from build123d import *

# Parameters (mm, degrees)
BOSS_EXTRUDE2_DEPTH = 100
SKETCH2_W           = 4.5
SKETCH2_H           = 54.5
BOSS_EXTRUDE3_DEPTH = 35
CHAMFER1_SIZE       = 3
DRAFT2_ANGLE        = 4


with BuildPart() as part:
    # Sketch1 → Boss-Extrude2 (new body)
    with BuildSketch(Plane(origin=(0, 0, 0), x_dir=(1, 0, 0), z_dir=(0, 1, 0))):
        Polygon((-31.066017178, -75), (31.066017178, -75), (75, -31.066017178), (75, 31.066017178), (31.066017178, 75), (-31.066017178, 75), (-75, 31.066017178), (-75, -31.066017178), align=None)
        Polygon((28.994949366, -70), (70, -28.994949366), (70, 28.994949366), (28.994949366, 70), (-28.994949366, 70), (-70, 28.994949366), (-70, -28.994949366), (-28.994949366, -70), align=None, mode=Mode.SUBTRACT)
    extrude(amount=BOSS_EXTRUDE2_DEPTH)

    # Sketch2 → Boss-Extrude3 (add)
    with BuildSketch(Plane.XY.offset(-70)):
        with Locations((-21.744949366, 27.25)):
            Rectangle(SKETCH2_W, SKETCH2_H)
        with Locations((3.755050634, 27.860857485)):
            Rectangle(SKETCH2_W, SKETCH2_H)
    extrude(amount=BOSS_EXTRUDE3_DEPTH)

    # Chamfer1
    chamfer1_edges = [part.edges().sort_by_distance(p)[0] for p in [
        (-31.066017178, 50, 75),
        (-75, 50, 31.066017178),
        (-75, 50, -31.066017178),
        (-31.066017178, 50, -75),
        (31.066017178, 50, -75),
        (75, 50, -31.066017178),
        (75, 50, 31.066017178),
        (31.066017178, 50, 75),
    ]]
    chamfer(chamfer1_edges, length=CHAMFER1_SIZE)

    # Draft2
    draft2_faces = [part.faces().sort_by_distance(p)[0] for p in [
        (53.033008589, 50, -53.033008589),
        (0, 50, -75),
        (-53.033008589, 50, -53.033008589),
        (-75, 50, 0),
        (-53.033008589, 50, 53.033008589),
        (0, 50, 75),
        (53.033008589, 50, 53.033008589),
        (75, 50, 0),
    ]]
    draft(draft2_faces, Plane.ZX.offset(100), DRAFT2_ANGLE)


solid = part.part
The model under review builds one solid part; all positions refer to its coordinate system, in mm. A direction names the side the tool comes from. Round coordinates to 2 decimals unless told otherwise and drop trailing zeros. Write each loop counter-clockwise with the first axis right and the second up, starting at its lowest first coordinate (ties: lowest second). Pieces come first, ordered by that corner, then holes. Notation, with made-up numbers: (51.5, 50.25) - (85.5, 50.25) arc R31 cw to (85.5, 77.25) - close; hole circle Ø2 at (67, -28). An arc over 180 degrees is marked (long way). One line per item, written item: value. Start each with the question number.
1. Consider section B-B on x = 24. Write out the cut boundary in (y, z), and give its area (3 significant figures).
2. Clearance check with flat-ended pins moving along their axes: P1, Ø5, axis at x = -23, z = -44.5, coming from the +Y side; P2, Ø17.5, axis at y = 30, z = -10, coming from the -X side; P3, Ø1.5, axis at x = 54.5, y = 60.5, coming from the +Z side. State where each tip first meets the part, or that it passes through.
3. Consider section A-A on z = -8.5. Write out the cut boundary in (x, y).
4. The part is to be moulded in two halves that separate along Z. For faces 3 (the face through (50, 100, 50)), 4 (the face through (30.899, 38.189, 73.827)), 5 (the face through (4, 55.111, -53)), say which applies: released by +Z, released by -Z, zero draft, split by the parting line, or undercut.
5. To check wall thickness, follow L1, parallel to X at y = 40.5, z = -56.5; L2, parallel to X at y = 16, z = -49.5; L3, parallel to X at y = 18.5, z = -33. State the ranges of each line that lie inside material, in increasing order. Write a range as from..to.
6. Machinability: for faces 1 (the face through (54.71, 60.41, 55.27)), 2 (the face through (49.21, 49.3, 49.785)), which of the approach directions +Z, -Z, +X, -X, +Y, -Y give a long, thin tool a straight path to every point of the face, cutting with its end or side? Answer none if there is none.
7. Consider section D-D on z = -38.5. Write out the cut boundary in (x, y).
Checks:
1. outline: (0, -76.68) - (75.91, -76.68) - (100, -75) - (100, -70) - (0, -70) - close; (0, 70) - (100, 70) - (100, 75) - (75.91, 76.68) - (0, 76.68) - close
1. area: 1,300 mm^2
2. P1: stops at y = 54.5
2. P2: stops at x = -80.51
2. P3: stops at z = 56.23
3. outline: (-81.99, 0) - (-70, 0) - (-70, 100) - (-75, 100) - close; (70, 0) - (81.99, 0) - (75, 100) - (70, 100) - close
4. face 3: zero draft
4. face 4: released by +Z
4. face 5: undercut
5. L1: x = -55.45..-42.49, -23.99..-19.49, 1.51..6.01, 42.49..55.45
5. L2: x = -64.87..-49.49, -23.99..-19.49, 1.51..6.01, 49.49..64.87
5. L3: x = -72.96..-65.99, 65.99..72.96
6. face 1: +Z, +X, +Y
6. face 2: +Y, -Y
7. outline: (-70.68, 0) - (-60.49, 0) - (-60.49, 100) - (-67.57, 100) - (-70.68, 68.53) - close; (-23.99, 0) - (-19.49, 0) - (-19.49, 54.5) - (-23.99, 54.5) - close; (1.51, 0.61) - (6.01, 0.61) - (6.01, 55.11) - (1.51, 55.11) - close; (60.49, 0) - (70.68, 0) - (70.68, 68.53) - (67.57, 100) - (60.49, 100) - close
